Print and shaded views of the part. All mm, measured from the part's lowest x, y and z. Round coordinates to 2 decimals unless told otherwise and drop trailing zeros. Loops run counter-clockwise (first coordinate to the right, second up) from the corner with the lowest first, then second, coordinate; pieces in that order, holes last. Notation, with made-up numbers: (26, -35) -> (45, -35) arc R29 cw to (45, -14) -> close; hole circle Ø5 at (-35, -11). An arc over 180 degrees is marked (long way). Answer as CSV lines item,"result".
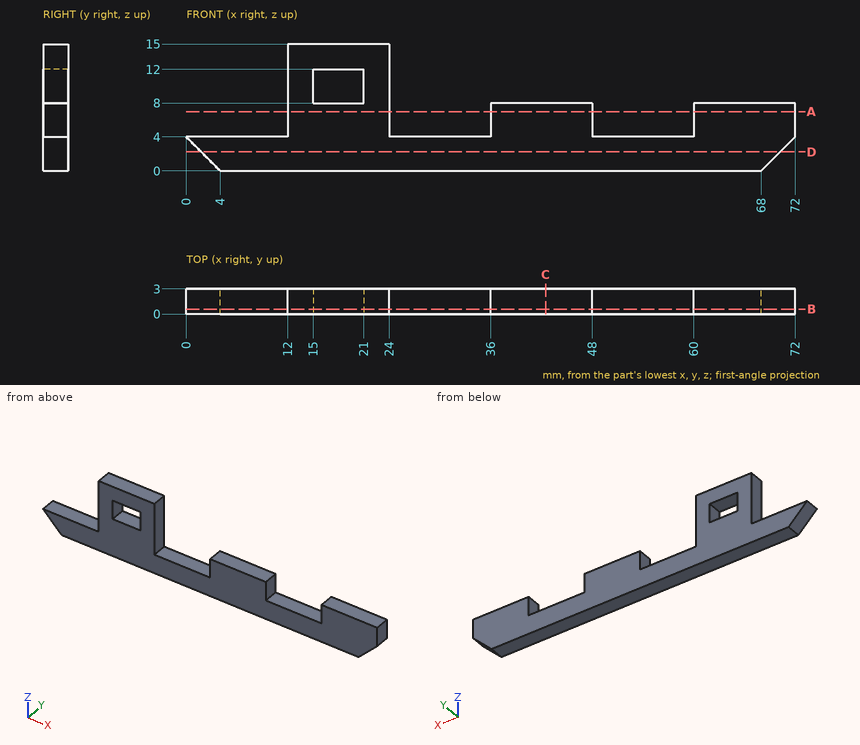
Q1. Saw through at C-C, the plane x = 42.5. Write the cut outline in (y, z), then the cut area to 3 significant figures.
Geometry results:
outline,"(0, 0) -> (3, 0) -> (3, 8) -> (0, 8) -> close"
area,"24.0 mm2"
Q2. Drill centre lines: line 1 along X through (y, z) = (0.7, 4.5); line 2 along Z through (x, y) = (20, 2.8); line 3 along X through (y, z) = (2.7, 11.5). Where is each one in solid material? Low to high.
Geometry results:
line 1,"12 to 24, 36 to 48, 60 to 72"
line 2,"0 to 8, 12 to 15"
line 3,"12 to 15, 21 to 24"
Q3. Drop flat-ended pins along their axis: P1, Ø0.9, axis at y = 1.5, z = 8.5, coming from the -X side; P2, Ø0.9, axis at y = 2, z = 9.5, coming from the +X side; P3, Ø0.9, axis at x = 30, y = 1.5, coming from the +Z side. Give the stop position or say it passes through.
Geometry results:
P1,"x = 12"
P2,"x = 24"
P3,"z = 4"
Q4. Saw through at B-B, the plane y = 0.6. Write the cut outline in (x, z).
Geometry results:
outline,"(0, 4) -> (4, 0) -> (68, 0) -> (72, 4) -> (72, 8) -> (60, 8) -> (60, 4) -> (48, 4) -> (48, 8) -> (36, 8) -> (36, 4) -> (24, 4) -> (24, 15) -> (12, 15) -> (12, 4) -> close; hole (15, 8) -> (21, 8) -> (21, 12) -> (15, 12) -> close"
Q5. Saw through at D-D, the plane z = 2.25. Write the cut outline in (x, y), then the cut area to 4 significant figures.
Geometry results:
outline,"(1.75, 0) -> (70.25, 0) -> (70.25, 3) -> (1.75, 3) -> close"
area,"205.5 mm2"
Q6. Saw through at A-A, the plane z = 7. Write the cut outline in (x, y), then the cut area to 3 significant figures.
Geometry results:
outline,"(12, 0) -> (24, 0) -> (24, 3) -> (12, 3) -> close; (36, 0) -> (48, 0) -> (48, 3) -> (36, 3) -> close; (60, 0) -> (72, 0) -> (72, 3) -> (60, 3) -> close"
area,"108 mm2"
